```python
from build123d import *

# Parameters (mm, degrees)
SKETCH1_W           = 79.375
SKETCH1_H           = 15.875
BOSS_EXTRUDE1_DEPTH = 7.9375
SKETCH2_R           = 4.7625
CUT_EXTRUDE1_DEPTH  = 19.05
SKETCH3_R           = 3.175
CUT_EXTRUDE2_DEPTH  = 44.475478002


with BuildPart() as part:
    # Sketch1 → Boss-Extrude1 (new, symmetric)
    with BuildSketch(Plane.XY):
        Rectangle(SKETCH1_W, SKETCH1_H)
    extrude(amount=BOSS_EXTRUDE1_DEPTH, both=True)

    # Sketch2 → Cut-Extrude1 (cut)
    with BuildSketch(Plane.ZY.offset(39.6875)):
        Circle(SKETCH2_R)
    extrude(amount=-CUT_EXTRUDE1_DEPTH, mode=Mode.SUBTRACT)

    # Sketch3 → Cut-Extrude2 (cut, through all)
    with BuildSketch(Plane(origin=(0, 7.9375, 0), x_dir=(1, 0, 0), z_dir=(0, 1, 0))):
        with Locations(Location((33.3375, 0, 0), (0, 0, 180))):
            Circle(SKETCH3_R)
        with Locations(Location((-11.1125, 0, 0), (0, 0, 180))):
            Circle(SKETCH3_R)
    extrude(amount=-CUT_EXTRUDE2_DEPTH, mode=Mode.SUBTRACT)


solid = part.part
```
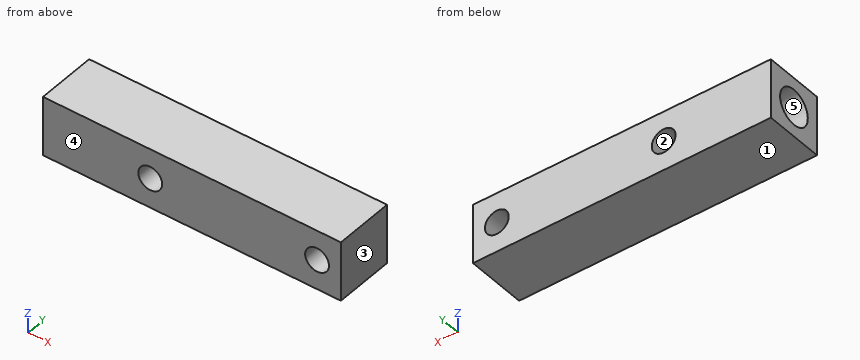
Model file for the job. Use its own axes, mm. Face numbers are marked on the shaded views. A direction names the side the tool comes from. Coordinates: 2 decimals unless noted, no trailing zeros. Loops run counter-clockwise (first coordinate to the right, second up) from the corner with the lowest first, then second, coordinate; pieces in that order, holes last. Notation, with made-up numbers: (21.5, 36.5) -> (63.5, 36.5) arc R6 ccw to (63.5, 47.5) -> close; hole circle Ø8 at (-28, -39). An arc over 180 degrees is marked (long way). Answer as a JSON object with one key per item and string values.
Q1. Probe probe 1 along X at (y, z) = (6, -0.25); probe 2 along Y at (x, z) = (-25.25, 0); probe 3 along X at (y, z) = (-3, -0.5). List the from-to ranges inside material, lowest first.
Report:
{"probe 1": "x = -39.69 to -14.28, -7.95 to 30.17, 36.5 to 39.69", "probe 2": "y = -7.94 to -4.76, 4.76 to 7.94", "probe 3": "x = -20.64 to -14.25, -7.98 to 30.2, 36.47 to 39.69"}
Q2. Cut at B-B (z = 0). List the corners of the cut face in (x, y).
Report:
{"outline": "(-39.69, -7.94) -> (-14.29, -7.94) -> (-14.29, 7.94) -> (-39.69, 7.94) -> (-39.69, 4.76) -> (-20.64, 4.76) -> (-20.64, -4.76) -> (-39.69, -4.76) -> close; (-7.94, -7.94) -> (30.16, -7.94) -> (30.16, 7.94) -> (-7.94, 7.94) -> close; (36.51, -7.94) -> (39.69, -7.94) -> (39.69, 7.94) -> (36.51, 7.94) -> close"}
Q3. Flat gauge pin, fed straight in: P1, Ø8.5, axis at x = 33.34, z = 0, coming from the +Y side. Where does the tip first touch, or does it go through?
Report:
{"P1": "stops at y = 7.94"}
Q4. Cut at A-A (y = 0). State how many separate pieces and enclosed holes the cut face has, and give its area (3 significant figures).
Report:
{"separate pieces": "1", "enclosed holes": "2", "area": "1,020 mm2"}
Q5. 3-axis set-ups, long thin cutter, end or side, ignore diameter. For the marked faces 4 and 5: which of +Z, -Z, +X, -X, +Y, -Y reach the whole face in a straight line?
Report:
{"face 4": "+Z, -Z, +X, -X, -Y", "face 5": "-X"}
Q6. Pull direction Z, two halves, no side cores. Call the marked faces 1, 2 and 3: released by +Z, released by -Z, zero draft, split by the parting line, or undercut.
Report:
{"face 1": "released by -Z", "face 2": "undercut", "face 3": "zero draft"}
Q7. Cut at C-C (x = 34). List the corners of the cut face in (y, z), and give its area (3 significant figures).
Report:
{"outline": "(-7.94, -7.94) -> (7.94, -7.94) -> (7.94, -3.11) -> (-7.94, -3.11) -> close; (-7.94, 3.11) -> (7.94, 3.11) -> (7.94, 7.94) -> (-7.94, 7.94) -> close", "area": "153 mm2"}
